For this review, take the finished solid that the model builds, in its own axes (mm). Round coordinates to 2 decimals unless told otherwise and drop trailing zeros. Loops run counter-clockwise (first coordinate to the right, second up) from the corner with the lowest first, then second, coordinate; pieces in that order, holes last.
1) Take a section at A-A (z = -12.25). State the section outline as (x, y) points.
2) Wall thickness on L1, parallel to Y at x = 12.3, z = -17.75; L2, parallel to Y at x = 12.45, z = -21.25; L3, parallel to Z at x = 13.2, y = -22: over which ranges is each line inside the solid? List them lowest first.
3) Take a section at B-B (z = -14). State the section outline as (x, y) points.
4) Insertion check: pin 1 (0.5 mm diameter, centred on y = -20.5, z = -21.5, fed in from +X); pin 2 (0.5 mm diameter, centred on x = 11, z = -21.5, fed in from -Y); pin 3 (1 mm diameter, centred on x = 12.5, z = -21.5, fed in from +Y). Each pin has a flat end and moves straight along its axis. Give the tip position at first contact, or say it passes through.
5) Mouldability with a two-part tool opening along Y and no side actions: class faces 1 (the conical face through (11.75, -20.62, -15.55)), 2 (the flat face through (12.5, -21.2, -21.7)), 3 (the flat face through (11.6, -21.4, -22)) as pulls with the +Y half, pulls with the -Y half, needs draft (parallel to the pull), parting line crosses it, or undercut.
```python
from build123d import *

# Parameters (mm, degrees)
POCKET005_DEPTH         = 0.2
POLARPATTERN005_COUNT   = 2
POLARPATTERN005_ANGLE   = 90
BODY009_PLACEMENT_ANGLE = 180


with BuildPart() as part:
    # Sketch017 → Revolution005 (revolve)
    with BuildSketch(Plane.XZ):
        Polygon((0, 0), (0, -12), (0.9, -1.05), (1.85, -0.1), (1.85, 0), align=None)
    revolve(axis=Axis((0, 0, 0), (0, 0, 1)))

    # Sketch018 → Pocket005 (cut, symmetric)
    with BuildSketch(Plane.XZ):
        Polygon((-1.15, 0), (0, -1.15), (1.15, 0), align=None)
    pocket005 = extrude(amount=POCKET005_DEPTH, both=True, mode=Mode.SUBTRACT)

    # PolarPattern005: Pocket005 ×2 about axis
    polarpattern005_axis = Axis((0, 0, 0), (0, 0, 1))
    for i in range(1, POLARPATTERN005_COUNT):
        add(pocket005.rotate(polarpattern005_axis, i * POLARPATTERN005_ANGLE / (POLARPATTERN005_COUNT - 1)), mode=Mode.SUBTRACT)


with BuildPart() as part_1:
    # Body009 placement: moved
    add(part.part.moved(Location((12, -21, -22))).rotate(Axis((12, -21, -22), (0, 1, 0)), BODY009_PLACEMENT_ANGLE))


solid = part_1.part
```
Response:
1. outline: circle Ø0.37 at (12, -21)
2. L1: y = -21.56 to -20.44
2. L2: y = -22.11 to -19.89
2. L3: z = -22 to -21.61
3. outline: circle Ø0.66 at (12, -21)
4. pin 1: stops at x = 13.63
4. pin 2: stops at y = -22.42
4. pin 3: stops at y = -19.16
5. face 1: parting line crosses it
5. face 2: undercut
5. face 3: needs draft
